Here's how the part is built. I have some questions about the finished solid (model axes, mm). Face numbers are marked on the shaded views. A direction names the side the tool comes from. Give positions to 0.01 mm unless a question says otherwise; leave off trailing zeros. Write each loop counter-clockwise with the first axis right and the second up, starting at its lowest first coordinate (ties: lowest second). Pieces come first, ordered by that corner, then holes. Notation, with made-up numbers: M 82.25,-35 L 136.25,-35 A19 ccw 136.25,-23 Z; hole C 0,60 d11. An arc over 180 degrees is marked long. Use one line per item in the form item = value. Start each with the question number.
from build123d import *

# Parameters (mm, degrees)
F1_DEPTH = 6
F2_R     = 3
F3_DEPTH = 25
F4_R     = 1.525
F5_DEPTH = 8


with BuildPart() as f1:
    # F0 (on Top) → F1 (new body)
    with BuildSketch(Plane.XY):
        with BuildLine():
            Line((-28.736944, 4), (-56.736944, 4))
            ThreePointArc((-56.736944, 4), (-59.565371, 2.828427), (-60.736944, 0))
            ThreePointArc((-60.736944, 0), (-59.565371, -2.828427), (-56.736944, -4))
            Line((-56.736944, -4), (-28.736944, -4))
            ThreePointArc((-28.736944, -4), (-25.908517, -2.828427), (-24.736944, 0))
            ThreePointArc((-24.736944, 0), (-25.908517, 2.828427), (-28.736944, 4))
        make_face()
        with BuildLine():
            ThreePointArc((-48.736944, 0), (-48.151158, 1.414214), (-46.736944, 2))
            Line((-46.736944, 2), (-30.736944, 2))
            ThreePointArc((-30.736944, 2), (-29.32273, 1.414214), (-28.736944, 0))
            ThreePointArc((-28.736944, 0), (-29.32273, -1.414214), (-30.736944, -2))
            Line((-30.736944, -2), (-46.736944, -2))
            ThreePointArc((-46.736944, -2), (-48.151158, -1.414214), (-48.736944, 0))
        make_face(mode=Mode.SUBTRACT)
    extrude(amount=F1_DEPTH)

    # F2 (on face) → F3 (join)
    with BuildSketch(Plane.XY.offset(6)):
        with Locations((-56.736944, 0)):
            Circle(F2_R)
    extrude(amount=F3_DEPTH)

    # F4 (on face) → F5 (cut)
    with BuildSketch(Plane.XY.offset(31)):
        with Locations((-56.736944, 0)):
            Circle(F4_R)
    extrude(amount=-F5_DEPTH, mode=Mode.SUBTRACT)


solid = f1.part
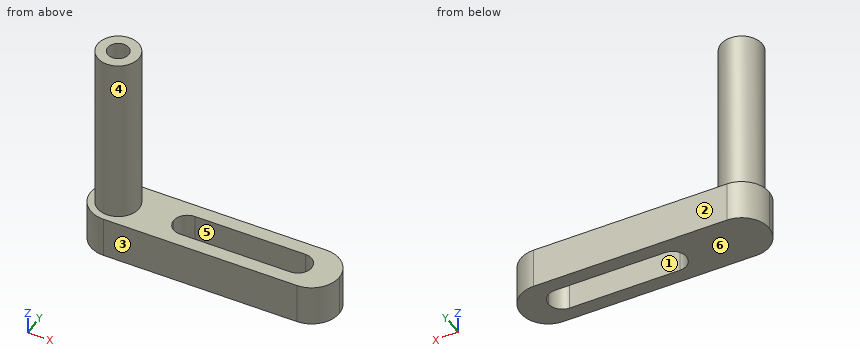
1) Suppose I cut it at D-D, the plane z = 21.5. List the corners of the cut face in (x, y) for me.
2) On a 3-axis mill with a long thin cutter (end or side, diameter ignored), from which of +Z, -Z, +X, -X, +Y, -Y can I reach the whole of each face in a straight line? I mean the marked faces 1 and 2. Say none if no direction works.
3) Thinking about a two-plate mould opening in Y: for the marked faces 3, 4, 5 and 6, which applies, released by +Y, released by -Y, zero draft, split by the parting line, or undercut?
4) Will these pins go through, and if not, where does the flat tip stop? P1, Ø1.5, axis at y = 2, z = 12, coming from the +X side; P2, Ø1, axis at x = -38.5, y = -1, coming from the +Z side; P3, Ø4, axis at x = -47.5, y = -2, coming from the +Z side.
5) Suppose I cut it at A-A, the plane x = -32. List the corners of the cut face in (y, z) for me, and give its area (3 significant figures).
6) Please list where these lines run through material, in increasing order: line 1 (Y direction, x = -35, z = 5.5); line 2 (Z direction, x = -56, y = -1.25); line 3 (Z direction, x = -50, y = 0.25).
7) Suppose I cut it at B-B, the plane y = -0.5. List the corners of the cut face in (x, z) for me, and give its area (3 significant figures).
8) Suppose I cut it at C-C, the plane z = 4.5. List the corners of the cut face in (x, y) for me.
Checks:
q1.outline = C -56.74,0 d6
q2.face_1 = +Z, -Z
q2.face_2 = +Z, -Z, +X, -X, +Y
q3.face_3 = released by -Y
q3.face_4 = split by the parting line
q3.face_5 = undercut
q3.face_6 = zero draft
q4.P1 = -54.01
q4.P2 = through
q4.P3 = 6
q5.outline = M -4,0 L -2,0 L -2,6 L -4,6 Z; M 2,0 L 4,0 L 4,6 L 2,6 Z
q5.area = 24.0 mm^2
q6.line_1 = -4 to -2, 2 to 4
q6.line_2 = 0 to 23
q6.line_3 = 0 to 6
q7.outline = M -60.71,0 L -48.67,0 L -48.67,6 L -53.78,6 L -53.78,31 L -55.3,31 L -55.3,23 L -58.18,23 L -58.18,31 L -59.69,31 L -59.69,6 L -60.71,6 Z; M -28.8,0 L -24.77,0 L -24.77,6 L -28.8,6 Z
q7.area = 221 mm^2
q8.outline = M -56.74,-4 L -28.74,-4 A4 ccw -28.74,4 L -56.74,4 A4 ccw Z; hole M -48.74,0 A2 ccw -46.74,-2 L -30.74,-2 A2 ccw -28.74,0 A2 ccw -30.74,2 L -46.74,2 A2 ccw Z
